Build history of the part. All positions in model axes, mm. A direction names the side the tool comes from. Round coordinates to 2 decimals unless told otherwise and drop trailing zeros. Write each loop counter-clockwise with the first axis right and the second up, starting at its lowest first coordinate (ties: lowest second). Pieces come first, ordered by that corner, then holes. Notation, with made-up numbers: (74, 16) -> (113, 16) arc R12 ccw to (113, 35) -> close; hole circle Ø7 at (54.5, 5.25). An arc over 180 degrees is marked (long way). Answer as CSV lines item,"result".
from build123d import *

# Parameters (mm, degrees)
SKETCH_1_W          = 200
SKETCH_1_H          = 100
EXTRUDE_1_DEPTH     = 70
SKETCH_3_R          = 20
CUT_EXTRUDE_1_DEPTH = 40
CUT_EXTRUDE_2_DEPTH = 40


with BuildPart() as part:
    # Sketch 1 → Extrude 1 (new body)
    with BuildSketch(Plane(origin=(0, 0, 0), x_dir=(1, 0, 0), z_dir=(0, 1, 0))):
        with Locations((100, 50)):
            Rectangle(SKETCH_1_W, SKETCH_1_H)
    extrude(amount=-EXTRUDE_1_DEPTH)

    # Sketch 3 → Cut-Extrude 1 (cut)
    with BuildSketch(Plane(origin=(0, 0, 0), x_dir=(1, 0, 0), z_dir=(0, 1, 0))):
        with Locations(Location((49.017273864, 50, 0), (0, 0, 270))):
            Circle(SKETCH_3_R)
    extrude(amount=-CUT_EXTRUDE_1_DEPTH, mode=Mode.SUBTRACT)

    # Sketch 3_3 → Cut-Extrude 2 (cut)
    with BuildSketch(Plane(origin=(0, 0, 0), x_dir=(1, 0, 0), z_dir=(0, 1, 0))):
        with BuildLine():
            ThreePointArc((170.982726136, 50), (150.982726136, 70), (130.982726136, 50))
            Line((130.982726136, 50), (170.982726136, 50))
        make_face()
        with BuildLine():
            Line((170.982726136, 50), (130.982726136, 50))
            ThreePointArc((130.982726136, 50), (150.982726136, 30), (170.982726136, 50))
        make_face()
    extrude(amount=-CUT_EXTRUDE_2_DEPTH, mode=Mode.SUBTRACT)


solid = part.part
1. Mould opens along X. For faces 3 (the flat face through (0, -35, -49)), 4 (the flat face through (151, -40, -50)), 5 (the flat face through (99, -70, -51)) say: +X half, -X half, draft (parallel to the pull), parting line (faces both ways), or undercut.
Results found:
face 3,"-X half"
face 4,"undercut"
face 5,"draft"
2. Cut at D-D, the plane x = 135.5. Write the cut outline in (y, z), then the cut area to 3 significant figures.
Results found:
outline,"(-70, -100) -> (0, -100) -> (0, -62.66) -> (-40, -62.66) -> (-40, -37.34) -> (0, -37.34) -> (0, 0) -> (-70, 0) -> close"
area,"5,990 mm2"
3. Drop a flat-ended pin along its axis: pin 1 Ø2 at (x, z) = (53, -54.5) entering from +Y. Give the stop position or say it passes through.
Results found:
pin 1,"stops at y = -40"
4. Cut at B-B, the plane x = 31. Write the cut outline in (y, z).
Results found:
outline,"(-70, -100) -> (0, -100) -> (0, -58.68) -> (-40, -58.68) -> (-40, -41.32) -> (0, -41.32) -> (0, 0) -> (-70, 0) -> close"
5. Cut at C-C, the plane y = -34.5. Write the cut outline in (x, z), then the cut area to 3 significant figures.
Results found:
outline,"(0, -100) -> (200, -100) -> (200, 0) -> (0, 0) -> close; hole circle Ø40 at (49.02, -50); hole circle Ø40 at (150.98, -50)"
area,"17,500 mm2"
6. Which spindle directions (+Z, -Z, +X, -X, +Y, -Y) get a long thin tool onto all of the face, cutting with end or side? Do faces 1 (the flat face through (49, -40, -50)), 2 (the flat face through (200, -35, -49)). Say none if no direction does.
Results found:
face 1,"+Y"
face 2,"+Z, -Z, +X, +Y, -Y"
7. Cut at A-A, the plane z = -50. Write the cut outline in (x, y).
Results found:
outline,"(0, -70) -> (200, -70) -> (200, 0) -> (170.98, 0) -> (170.98, -40) -> (130.98, -40) -> (130.98, 0) -> (69.02, 0) -> (69.02, -40) -> (29.02, -40) -> (29.02, 0) -> (0, 0) -> close"
8. Probe line 1 along X through (y, z) = (-21, -49); line 2 along X through (y, z) = (-20, -67); line 3 along Z through (x, y) = (61, -14.5). List the from-to ranges inside material, lowest first.
Results found:
line 1,"x = 0 to 29.04, 68.99 to 131.01, 170.96 to 200"
line 2,"x = 0 to 38.48, 59.55 to 140.45, 161.52 to 200"
line 3,"z = -100 to -66.01, -33.99 to 0"
